Part model, mm, in its own coordinate system. Face numbers are marked on the shaded views. A direction names the side the tool comes from. Give positions to 0.01 mm unless a question says otherwise; leave off trailing zeros. Write each loop counter-clockwise with the first axis right and the second up, starting at its lowest first coordinate (ties: lowest second). Pieces come first, ordered by that corner, then holes. Notation, with made-up numbers: M -10.75,12.5 L 0.25,12.5 A27 cw 0.25,45.5 Z; hole C 79,75 d2. An arc over 180 degrees is marked long. Answer as CSV lines item,"result". Start each with the question number.
1) Slice it at A-A, the plane x = 16. Give the cut face in (y, z).
2) Tool access for the marked faces 1, 2 and 3: list every direction of +Z, -Z, +X, -X, +Y, -Y with a clear straight run to the whole face (end or side of a thin tool).
3) Wall check: line 1 along Z through (x, y) = (16.5, 10.75); line 2 along X through (y, z) = (4.75, -47); line 3 along Y through (x, z) = (30.5, -46). Give the ranges that are in metal, low to high. Write a range as from..to.
4) Slice it at B-B, the plane z = -42. Give the cut face in (x, y), plus the area to 3 significant figures.
5) Slice it at C-C, the plane y = 6. Give the cut face in (x, z).
6) Pin check, flat tips, straight feed: pin 1 Ø1 at (y, z) = (9, -6) entering from -X; pin 2 Ø3.5 at (x, z) = (20, -41) entering from -Y; pin 3 Ø2.5 at (y, z) = (3.5, -44.5) entering from +X. Stop position of each tip, or through.
7) Slice it at D-D, the plane z = -35. Give the cut face in (x, y), plus the area to 3 significant figures.
```python
from build123d import *

# Parameters (mm, degrees)
BOSS_EXTRUDE2_DEPTH = 37
BOSS_EXTRUDE3_DEPTH = 12


with BuildPart() as part:
    # Sketch1 → Boss-Extrude2 (new body)
    with BuildSketch(Plane.XY):
        with BuildLine():
            Line((6, 0), (41, 0))
            ThreePointArc((41, 0), (47, 6), (41, 12))
            Line((41, 12), (6, 12))
            ThreePointArc((6, 12), (0, 6), (6, 0))
        make_face()
    extrude(amount=-BOSS_EXTRUDE2_DEPTH)

    # Sketch2 → Boss-Extrude3 (add)
    with BuildSketch(Plane(origin=(0, 0, -37), x_dir=(-1, 0, 0), z_dir=(0, 0, -1))):
        with BuildLine():
            Line((-42.5, 2), (-4.5, 2))
            Line((-4.5, 2), (-4.5, 7))
            ThreePointArc((-4.5, 7), (-5.085786438, 8.414213562), (-6.5, 9))
            Line((-6.5, 9), (-40.5, 9))
            ThreePointArc((-40.5, 9), (-41.914213562, 8.414213562), (-42.5, 7))
            Line((-42.5, 7), (-42.5, 2))
        make_face()
    extrude(amount=BOSS_EXTRUDE3_DEPTH)


solid = part.part
```
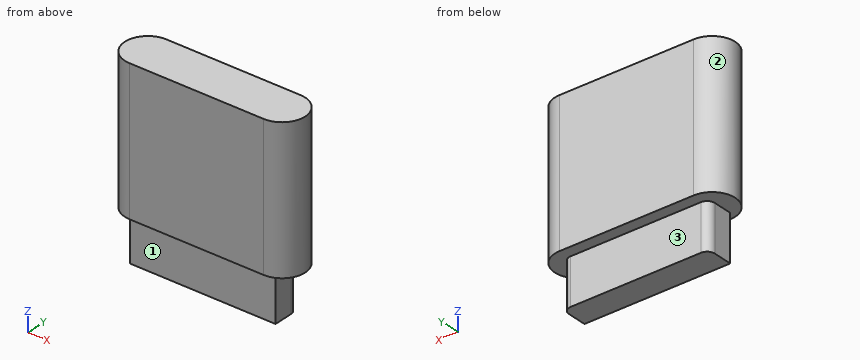
Found:
1,outline,"M 0,-37 L 2,-37 L 2,-49 L 9,-49 L 9,-37 L 12,-37 L 12,0 L 0,0 Z"
2,face 1,"-Z, +X, -X, -Y"
2,face 2,"+Z, -Z, -X"
2,face 3,"-Z, +X, -X, +Y"
3,line 1,"-37..0"
3,line 2,"4.5..42.5"
3,line 3,"2..9"
4,outline,"M 4.5,2 L 42.5,2 L 42.5,7 A2 ccw 40.5,9 L 6.5,9 A2 ccw 4.5,7 Z"
4,area,"264 mm²"
5,outline,"M 0,-37 L 4.5,-37 L 4.5,-49 L 42.5,-49 L 42.5,-37 L 47,-37 L 47,0 L 0,0 Z"
6,pin 1,"x = 0.55"
6,pin 2,"y = 2"
6,pin 3,"x = 42.5"
7,outline,"M 6,0 L 41,0 A6 ccw 41,12 L 6,12 A6 ccw Z"
7,area,"533 mm²"
